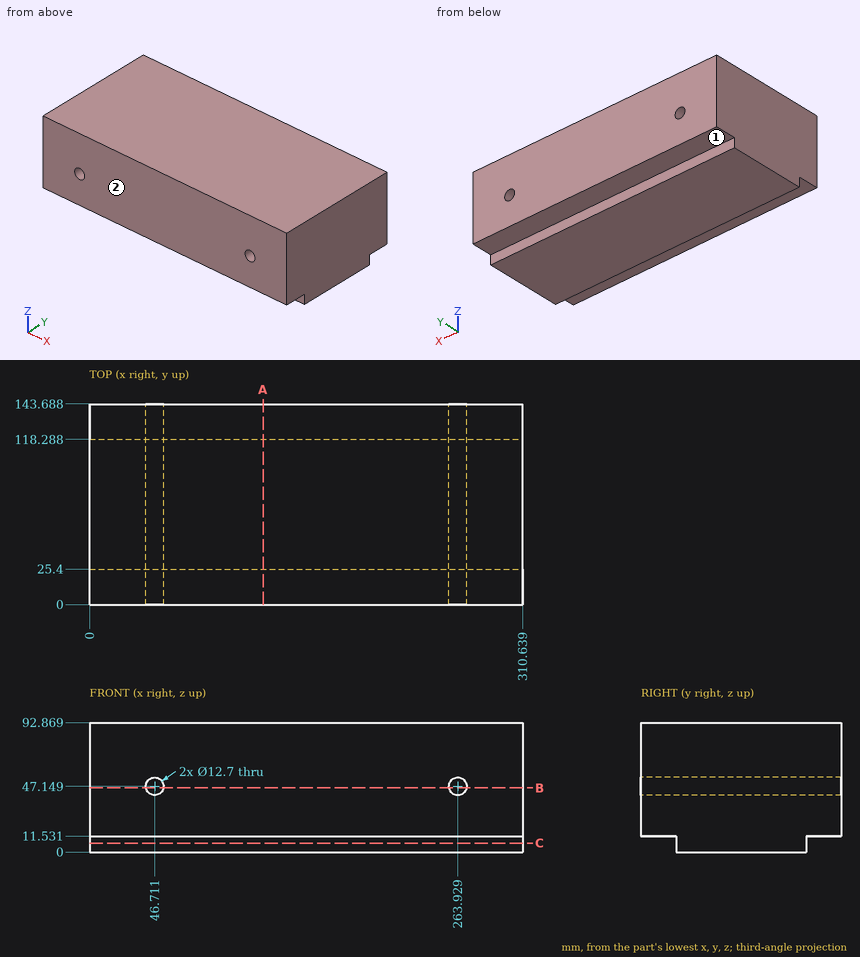
Here's the drawing with two shaded views (mm, measured from the low corner). I have some questions. A direction names the side the tool comes from. Coordinates: 2 decimals unless noted, no trailing zeros. Order: outer loops, then holes, each group sorted by start corner. A loop starts at its lowest first (then second) coordinate and runs counter-clockwise, first axis right, second up.
Item 1: Which directions (+Z, -Z, +X, -X, +Y, -Y) give clear straight access to the entire face, cutting with the end or side of a thin tool? Please do the marked faces 1 and 2.
Response values:
face 1: -Z, +X, -X, +Y
face 2: +Z, -Z, +X, -X, -Y
Item 2: If we section it at C-C, the plane z = 6.5: List the corners of the cut face in (x, y) for me, then the cut area to 3 significant figures.
Response values:
outline: (0, 25.4) - (310.64, 25.4) - (310.64, 118.29) - (0, 118.29) - close
area: 28,900 mm2
Item 3: I need wall thicknesses on probe 1 along X at (y, z) = (107, 45.5); probe 2 along X at (y, z) = (113.5, 52) (1 decimal); probe 3 along Z at (x, y) = (285, 137.5). Which ranges of each line are inside material? Lowest first, please.
Response values:
probe 1: x = 0 to 40.58, 52.84 to 257.8, 270.06 to 310.64
probe 2: x = 0 to 42.6, 50.8 to 259.8, 268 to 310.6
probe 3: z = 11.53 to 92.87
Item 4: If we section it at B-B, the plane z = 46: List the corners of the cut face in (x, y) for me (1 decimal), then the cut area to 3 significant figures.
Response values:
outline: (0, 0) - (40.5, 0) - (40.5, 143.7) - (0, 143.7) - close; (53, 0) - (257.7, 0) - (257.7, 143.7) - (53, 143.7) - close; (270.2, 0) - (310.6, 0) - (310.6, 143.7) - (270.2, 143.7) - close
area: 41,000 mm2
Item 5: I'm going to push flat-ended pins straight in: pin 1 Ø3.5 at (x, z) = (173, 3.5) entering from -Y; pin 2 Ø7.5 at (x, y) = (196.5, 126) entering from -Z. Where does each tip first touch, or does it pass through?
Response values:
pin 1: stops at y = 25.4
pin 2: stops at z = 11.53
Item 6: If we section it at A-A, the plane x = 124.5: List the corners of the cut face in (y, z) for me.
Response values:
outline: (0, 11.53) - (25.4, 11.53) - (25.4, 0) - (118.29, 0) - (118.29, 11.53) - (143.69, 11.53) - (143.69, 92.87) - (0, 92.87) - close
